Check sheet for the modelled part. Datum: model origin and axes. Units: mm. Face numbers are marked on the shaded views. A direction names the side the tool comes from. Round coordinates to 2 decimals unless told otherwise and drop trailing zeros. Order: outer loops, then holes, each group sorted by start corner. A loop starts at its lowest first (then second) coordinate and runs counter-clockwise, first axis right, second up.
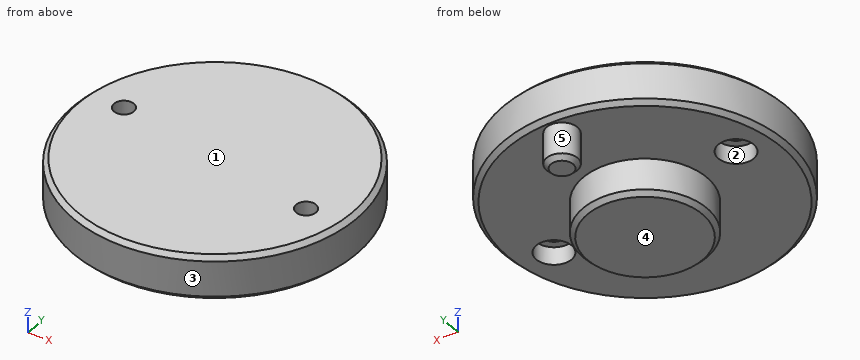
from build123d import *

# Parameters (mm, degrees)
SKETCH_1_R          = 3.5
EXTRUDE_1_DEPTH     = 5
FILLET_1_R          = 10
SKETCH_2_R          = 18
EXTRUDE_2_DEPTH     = 3
SKETCH_3_R          = 14
CUT_EXTRUDE_1_DEPTH = 32
SKETCH_4_R          = 16.75
CUT_EXTRUDE_2_DEPTH = 3
CHAMFER_1_SIZE      = 0.5
SKETCH_5_R          = 32
EXTRUDE_3_DEPTH     = 10
SKETCH_6_R          = 3.5
SKETCH_6_R_2        = 14
EXTRUDE_4_DEPTH     = 8
SKETCH_7_W          = 21.874500366
SKETCH_7_H          = 73.978344987
CUT_EXTRUDE_3_DEPTH = 62.5
CHAMFER_2_SIZE      = 1
CHAMFER_3_SIZE      = 1
SKETCH_8_R          = 2.25
CUT_EXTRUDE_4_DEPTH = 125
SKETCH_9_R          = 4
CUT_EXTRUDE_5_DEPTH = 4


with BuildPart() as part:
    # 草图1 → 凸台-拉伸1 (new body)
    with BuildSketch(Plane.XY):
        with BuildLine():
            Line((-11.5, 18.165902125), (-7.564716302, 29.602895938))
            ThreePointArc((-7.564716302, 29.602895938), (0, 35), (7.564716302, 29.602895938))
            Line((7.564716302, 29.602895938), (11.5, 18.165902125))
            ThreePointArc((11.5, 18.165902125), (18.619546181, 10.75), (21.482132723, 0.876341081))
            Line((21.482132723, 0.876341081), (29.419218059, -8.250211479))
            ThreePointArc((29.419218059, -8.250211479), (30.310889132, -17.5), (21.854501757, -21.352684459))
            Line((21.854501757, -21.352684459), (9.982132723, -19.042243206))
            ThreePointArc((9.982132723, -19.042243206), (0, -21.5), (-9.982132723, -19.042243206))
            Line((-9.982132723, -19.042243206), (-21.854501757, -21.352684459))
            ThreePointArc((-21.854501757, -21.352684459), (-30.310889132, -17.5), (-29.419218059, -8.250211479))
            Line((-29.419218059, -8.250211479), (-21.482132723, 0.876341081))
            ThreePointArc((-21.482132723, 0.876341081), (-18.619546181, 10.75), (-11.5, 18.165902125))
        make_face()
        with Locations((0, 27)):
            Circle(SKETCH_1_R, mode=Mode.SUBTRACT)
        with Locations((23.382685902, -13.5)):
            Circle(SKETCH_1_R, mode=Mode.SUBTRACT)
        with Locations((-23.382685902, -13.5)):
            Circle(SKETCH_1_R, mode=Mode.SUBTRACT)
    extrude(amount=EXTRUDE_1_DEPTH)

    # 圆角1
    fillet_1_edges = [part.edges().sort_by_distance(p)[0] for p in [
        (21.482132723, 0.876341081, 2.5),
        (9.982132723, -19.042243206, 2.5),
        (-9.982132723, -19.042243206, 2.5),
        (-21.482132723, 0.876341081, 2.5),
        (-11.5, 18.165902125, 2.5),
        (11.5, 18.165902125, 2.5),
    ]]
    fillet(fillet_1_edges, radius=FILLET_1_R)

    # 草图2 → 凸台-拉伸2 (add)
    with BuildSketch(Plane.XY.offset(5)):
        Circle(SKETCH_2_R)
    extrude(amount=EXTRUDE_2_DEPTH)

    # 草图3 → 切除-拉伸1 (cut)
    with BuildSketch(Plane.XY.offset(8)):
        Circle(SKETCH_3_R)
    extrude(amount=-CUT_EXTRUDE_1_DEPTH, mode=Mode.SUBTRACT)

    # 草图4 → 切除-拉伸2 (cut)
    with BuildSketch(Plane(origin=(0, 0, 0), x_dir=(-1, 0, 0), z_dir=(0, 0, -1))):
        Circle(SKETCH_4_R)
    extrude(amount=-CUT_EXTRUDE_2_DEPTH, mode=Mode.SUBTRACT)

    # 倒角1
    chamfer_1_edges = [part.edges().sort_by_distance(p)[0] for p in [
        (-18, 0, 8),
    ]]
    chamfer(chamfer_1_edges, length=CHAMFER_1_SIZE)

    # 草图7 → 切除-拉伸3 (cut, symmetric)
    with BuildSketch(Plane(origin=(0, 0, 0), x_dir=(0, 0, -1), z_dir=(1, 0, 0))):
        with Locations((-1.024921742, 9.171265754)):
            Rectangle(SKETCH_7_W, SKETCH_7_H)
    extrude(amount=CUT_EXTRUDE_3_DEPTH, both=True, mode=Mode.SUBTRACT)


with BuildPart() as body_2:
    # 草图5 → 凸台-拉伸3 (new body)
    with BuildSketch(Plane.XY.offset(8)):
        Circle(SKETCH_5_R)
    extrude(amount=EXTRUDE_3_DEPTH)

    # 草图6 → 凸台-拉伸4 (add)
    with BuildSketch(Plane(origin=(0, 0, 8), x_dir=(-1, 0, 0), z_dir=(0, 0, -1))):
        with Locations(Location((0, 27, 0), (0, 0, 180))):
            Circle(SKETCH_6_R)
        with Locations(Location((0, 0, 0), (0, 0, 180))):
            Circle(SKETCH_6_R_2)
    extrude(amount=EXTRUDE_4_DEPTH)

    # 倒角2
    chamfer_2_edges = [body_2.edges().sort_by_distance(p)[0] for p in [
        (-3.5, 27, 0),
        (-14, 0, 0),
    ]]
    chamfer(chamfer_2_edges, length=CHAMFER_2_SIZE)

    # 倒角3
    chamfer_3_edges = [body_2.edges().sort_by_distance(p)[0] for p in [
        (-32, 0, 8),
        (-32, 0, 18),
    ]]
    chamfer(chamfer_3_edges, length=CHAMFER_3_SIZE)

    # 草图8 → 切除-拉伸4 (cut)
    with BuildSketch(Plane(origin=(0, 0, 8), x_dir=(-1, 0, 0), z_dir=(0, 0, -1))):
        with Locations((-23.210676004, -3.676209928)):
            Circle(SKETCH_8_R)
        with Locations(Location((23.210676004, 3.676209928, 0), (0, 0, 180))):
            Circle(SKETCH_8_R)
    extrude(amount=-CUT_EXTRUDE_4_DEPTH, mode=Mode.SUBTRACT)

    # 草图9 → 切除-拉伸5 (cut)
    with BuildSketch(Plane(origin=(0, 0, 8), x_dir=(-1, 0, 0), z_dir=(0, 0, -1))):
        with Locations((-23.210676004, -3.676209928)):
            Circle(SKETCH_9_R)
        with Locations((23.210676004, 3.676209928)):
            Circle(SKETCH_9_R)
    extrude(amount=-CUT_EXTRUDE_5_DEPTH, mode=Mode.SUBTRACT)


solid = body_2.part
1) Sectioned sample at C-C on z = 16.25. Record the cut outline in (x, y), and give its area (3 significant figures).
2) Draft check along Y on the marked faces 3, 4 and 5. Enter one of: pulls with the +Y half, pulls with the -Y half, needs draft (parallel to the pull), parting line crosses it, or undercut.
3) Gauge pin test, flat ends, axial feed: pin 1 (6 mm diameter, centred on y = -4, z = 13.5, fed in from -X); pin 2 (10 mm diameter, centred on x = 20.5, z = 16, fed in from +Y); pin 3 (2 mm diameter, centred on x = 24.5, z = 12, fed in from +Y); pin 4 (4 mm diameter, centred on x = -23.21, y = 3.68, fed in from +Z). Record the tip position at first contact, or that the pin passes through.
4) Sectioned sample at D-D on z = 11.25. Record the cut outline in (x, y), and give its area (3 significant figures).
5) Scan lines: line 1 (X direction, y = 0.5, z = 4.5); line 2 (Z direction, x = 21, y = 8); line 3 (Z direction, x = 24, y = -6). Record each from-to range of solid material in increasing order.
6) Set-up check for the marked faces 1 and 2: record each of +Z, -Z, +X, -X, +Y, -Y from which the full face is reachable in a straight line by a thin tool's end or side.
7) Sectioned sample at B-B on z = 5.5. Record the cut outline in (x, y).
8) Sectioned sample at A-A on x = 0. Record the cut outline in (y, z).
Values found:
1. outline: circle Ø64 at (0, 0); hole circle Ø4.5 at (-23.21, 3.68); hole circle Ø4.5 at (23.21, -3.68)
1. area: 3,190 mm2
2. face 3: parting line crosses it
2. face 4: needs draft
2. face 5: undercut
3. pin 1: stops at x = -31.98
3. pin 2: stops at y = 28
3. pin 3: stops at y = 21.72
3. pin 4: passes through
4. outline: circle Ø64 at (0, 0); hole circle Ø8 at (-23.21, 3.68); hole circle Ø8 at (23.21, -3.68)
4. area: 3,120 mm2
5. line 1: x = -13.99 to 13.99
5. line 2: z = 8 to 18
5. line 3: z = 12 to 18
6. face 1: +Z, +X, -X, +Y, -Y
6. face 2: -Z
7. outline: circle Ø28 at (0, 0); circle Ø7 at (0, 27)
8. outline: (-32, 9) - (-31, 8) - (-14, 8) - (-14, 1) - (-13, 0) - (13, 0) - (14, 1) - (14, 8) - (23.5, 8) - (23.5, 1) - (24.5, 0) - (29.5, 0) - (30.5, 1) - (30.5, 8) - (31, 8) - (32, 9) - (32, 17) - (31, 18) - (-31, 18) - (-32, 17) - close
